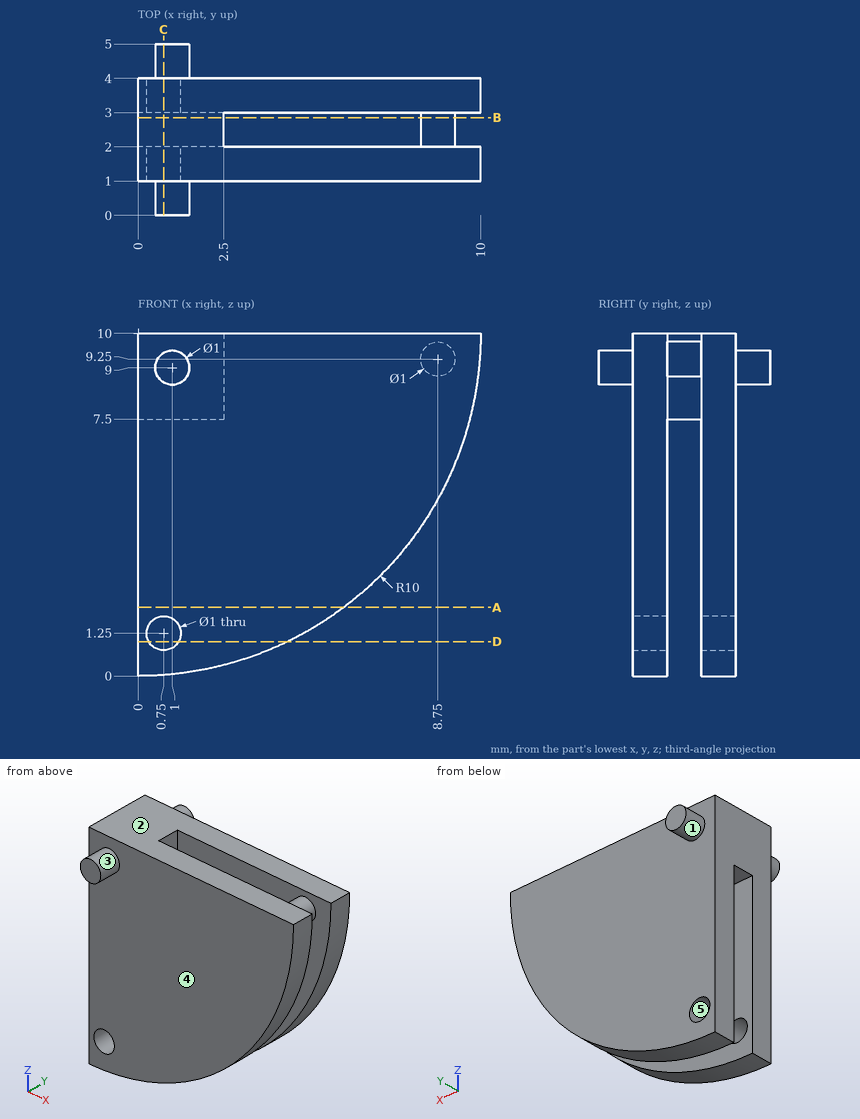
Design review of the part shown in the three views and the two pictorial views. Dimensions are in mm from the part's minimum x, y and z. A direction names the side the tool comes from. Coordinates: 2 decimals unless noted, no trailing zeros. Loops run counter-clockwise (first coordinate to the right, second up) from the corner with the lowest first, then second, coordinate; pieces in that order, holes last. Notation, with made-up numbers: (68, 0.25) - (78, 0.25) arc R15 cw to (78, 15.25) - close; hole circle Ø9 at (-31.75, -38). An arc over 180 degrees is marked (long way). Use a Markdown table: item, result. Add a question column.
Item 1: We need section D-D (z = 1). Give the boundary of the cut face in (x, y), and give its area (3 significant figures).
Item 2: Insertion check: pin 1 Ø1.5 at (x, z) = (8, 1.5) entering from -Y; pin 2 Ø0.5 at (y, z) = (2.5, 9.5) entering from +X; pin 3 Ø4 at (x, z) = (1, 4) entering from -Y; pin 4 Ø1.1 at (x, y) = (1, 2.5) entering from -Z. Each pin has a flat end and moves straight along its axis. Give the tip position at first contact, or say it passes through.
Item 3: Tool access review of the marked faces 1 and 2: name each direction out of +Z, -Z, +X, -X, +Y, -Y from which nothing blocks a thin tool from reaching the whole face with its end or side.
Item 4: We need section C-C (x = 0.75). Give the boundary of the cut face in (y, z), and give its area (3 significant figures).
Item 5: For line 1 (Y direction, x = 4.75, z = 1.5); line 2 (X direction, y = 2.3, z = 8); line 3 (Z direction, x = 1.75, y = 2.4), list the stretches that pass through material, from the lowest coordinate up.
Item 6: We need section B-B (y = 2.85). Give the boundary of the cut face in (x, z).
Item 7: We need section A-A (z = 2). Give the boundary of the cut face in (x, y).
Item 8: Mouldability with a two-part tool opening along X and no side actions: class the marked faces 3, 4 and 5 as pulls with the +X half, pulls with the -X half, needs draft (parallel to the pull), parting line crosses it, or undercut.
Results list:
| question | item | result |
|---|---|---|
| 1 | outline | (0, 1) - (0.32, 1) - (0.32, 2) - (0, 2) - close; (0, 3) - (0.32, 3) - (0.32, 4) - (0, 4) - close; (1.18, 1) - (4.36, 1) - (4.36, 2) - (1.18, 2) - close; (1.18, 3) - (4.36, 3) - (4.36, 4) - (1.18, 4) - close |
| 1 | area | 6.99 mm^2 |
| 2 | pin 1 | passes through |
| 2 | pin 2 | stops at x = 9.25 |
| 2 | pin 3 | stops at y = 1 |
| 2 | pin 4 | stops at z = 0.03 |
| 3 | face 1 | +Y |
| 3 | face 2 | +Z, +X, -X, +Y, -Y |
| 4 | outline | (0, 8.57) - (1, 8.57) - (1, 1.75) - (2, 1.75) - (2, 7.5) - (3, 7.5) - (3, 1.75) - (4, 1.75) - (4, 8.57) - (5, 8.57) - (5, 9.43) - (4, 9.43) - (4, 10) - (1, 10) - (1, 9.43) - (0, 9.43) - close; (1, 0.03) - (2, 0.03) - (2, 0.75) - (1, 0.75) - close; (3, 0.03) - (4, 0.03) - (4, 0.75) - (3, 0.75) - close |
| 4 | area | 22.2 mm^2 |
| 5 | line 1 | y = 1 to 2, 3 to 4 |
| 5 | line 2 | x = 0 to 2.5 |
| 5 | line 3 | z = 7.5 to 10 |
| 6 | outline | (0, 7.5) - (2.5, 7.5) - (2.5, 10) - (0, 10) - close; circle Ø1 at (8.75, 9.25) |
| 7 | outline | (0, 1) - (6, 1) - (6, 2) - (0, 2) - close; (0, 3) - (6, 3) - (6, 4) - (0, 4) - close |
| 8 | face 3 | parting line crosses it |
| 8 | face 4 | needs draft |
| 8 | face 5 | undercut |
